```python
from build123d import *

# Parameters (mm, degrees)
BOSS_EXTRUDE1_DEPTH     = 0.8
CUT_EXTRUDE1_DEPTH      = 145.88389317
CUT_EXTRUDE2_DEPTH      = 145.88389317
MIRROR2_COPY_1_DEPTH    = 145.88389317
FILLET1_R               = 5
SKETCH4_R               = 3.65
BOSS_EXTRUDE4_DEPTH     = 3
CUT_EXTRUDE5_DEPTH      = 145.931509686
CUT_EXTRUDE5_DEPTH_BACK = 145.931509686
SKETCH2_4_R             = 1.8
CUT_EXTRUDE6_DEPTH      = 2.2
CUT_EXTRUDE6_DEPTH_BACK = 145.912740986
SKETCH4_4_R             = 2.85


with BuildPart() as part:
    # Sketch1 → Boss-Extrude1 (new body)
    with BuildSketch(Plane.XY):
        Polygon((85.45, 117), (-85.45, 117), (-85.45, 107.6), (-52.367829575, 50.3), (-85.45, -7), (-85.45, -15.5), (85.45, -15.5), (85.45, -7), (52.367829575, 50.3), (85.45, 107.6), align=None)
    extrude(amount=-BOSS_EXTRUDE1_DEPTH)

    # Sketch1_3 → Cut-Extrude1 (cut, through all)
    with BuildSketch(Plane.XY):
        Polygon((67.078361679, 85.779389009), (73.377429493, 96.689694505), (67.078361679, 107.6), (54.480226049, 107.6), (48.181158234, 96.689694505), (54.480226049, 85.779389009), align=None)
        Polygon((57.892542518, 69.869083514), (51.593474703, 80.779389009), (38.995339074, 80.779389009), (32.696271259, 69.869083514), (38.995339074, 58.958778018), (51.593474703, 58.958778018), align=None)
        Polygon((27.696271259, 69.869083514), (21.397203444, 80.779389009), (8.799067815, 80.779389009), (2.5, 69.869083514), (8.799067815, 58.958778018), (21.397203444, 58.958778018), align=None)
        Polygon((36.88209042, 85.779389009), (43.181158234, 96.689694505), (36.88209042, 107.6), (24.28395479, 107.6), (17.984886975, 96.689694505), (24.28395479, 85.779389009), align=None)
    cut_extrude1 = extrude(amount=-CUT_EXTRUDE1_DEPTH, mode=Mode.SUBTRACT)

    # Sketch1_4 → Cut-Extrude2 (cut, through all)
    with BuildSketch(Plane.XY):
        Polygon((-6.299067815, 107.6), (-12.598135629, 96.689694505), (-6.299067815, 85.779389009), (6.299067815, 85.779389009), (12.598135629, 96.689694505), (6.299067815, 107.6), align=None)
    cut_extrude2 = extrude(amount=-CUT_EXTRUDE2_DEPTH, mode=Mode.SUBTRACT)

    # Mirror1: Cut-Extrude1 across plane
    add(cut_extrude1.mirror(Plane(origin=(0, 0, 0), x_dir=(0, 0, 1), z_dir=(1, 0, 0))), mode=Mode.SUBTRACT)

    # Mirror2: Cut-Extrude1, Cut-Extrude2 across plane
    add(cut_extrude1.mirror(Plane(origin=(0, 50.3, 0), x_dir=(0, 0, 1), z_dir=(0, -1, 0))), mode=Mode.SUBTRACT)
    add(cut_extrude2.mirror(Plane(origin=(0, 50.3, 0), x_dir=(0, 0, 1), z_dir=(0, -1, 0))), mode=Mode.SUBTRACT)

    # Mirror2 copy 1 sketch → Mirror2 copy 1 (cut, through all)
    with BuildSketch(Plane(origin=(0, 100.6, 0), x_dir=(-1, 0, 0), z_dir=(0, 0, 1))):
        Polygon((67.078361679, 85.779389009), (73.377429493, 96.689694505), (67.078361679, 107.6), (54.480226049, 107.6), (48.181158234, 96.689694505), (54.480226049, 85.779389009), align=None)
        Polygon((57.892542518, 69.869083514), (51.593474703, 80.779389009), (38.995339074, 80.779389009), (32.696271259, 69.869083514), (38.995339074, 58.958778018), (51.593474703, 58.958778018), align=None)
        Polygon((27.696271259, 69.869083514), (21.397203444, 80.779389009), (8.799067815, 80.779389009), (2.5, 69.869083514), (8.799067815, 58.958778018), (21.397203444, 58.958778018), align=None)
        Polygon((36.88209042, 85.779389009), (43.181158234, 96.689694505), (36.88209042, 107.6), (24.28395479, 107.6), (17.984886975, 96.689694505), (24.28395479, 85.779389009), align=None)
    extrude(amount=-MIRROR2_COPY_1_DEPTH, mode=Mode.SUBTRACT)

    # Fillet1
    fillet1_edges = [part.edges().sort_by_distance(p)[0] for p in [
        (85.45, 117, -0.4),
        (-85.45, 117, -0.4),
        (-85.45, -15.5, -0.4),
        (85.45, -15.5, -0.4),
    ]]
    fillet(fillet1_edges, radius=FILLET1_R)

    # Sketch4 → Boss-Extrude4 (add)
    with BuildSketch(Plane.XY):
        with Locations(Location((-78, -11.829016319, 0), (0, 0, 180))):
            Circle(SKETCH4_R)
        with Locations(Location((78, 112.3, 0), (0, 0, 180))):
            Circle(SKETCH4_R)
    extrude(amount=BOSS_EXTRUDE4_DEPTH)

    # Sketch2_4 → Cut-Extrude5 (cut, two sides: drawn at the far end of the back side and taken through both)
    with BuildSketch(Plane(origin=(0, 0, -0.8), x_dir=(-1, 0, 0), z_dir=(0, 0, -1)).offset(-CUT_EXTRUDE5_DEPTH_BACK)):
        with Locations((-78, 112.3)):
            Circle(SKETCH2_4_R)
        with Locations((78, -11.829016319)):
            Circle(SKETCH2_4_R)
    extrude(amount=CUT_EXTRUDE5_DEPTH + CUT_EXTRUDE5_DEPTH_BACK, mode=Mode.SUBTRACT)

    # Sketch4_4 → Cut-Extrude6 (cut, two sides: drawn at the far end of the back side and taken through both)
    with BuildSketch(Plane.XY.offset(-CUT_EXTRUDE6_DEPTH_BACK)):
        with Locations((-78, -11.829016319)):
            Circle(SKETCH4_4_R)
        with Locations((78, 112.3)):
            Circle(SKETCH4_4_R)
    extrude(amount=CUT_EXTRUDE6_DEPTH + CUT_EXTRUDE6_DEPTH_BACK, mode=Mode.SUBTRACT)


solid = part.part
```
Geometry check sheet. Reference: the model listing, model coordinates, mm. A direction names the side the tool comes from. Give positions to 0.01 mm unless a question says otherwise; leave off trailing zeros. Write each loop counter-clockwise with the first axis right and the second up, starting at its lowest first coordinate (ties: lowest second). Pieces come first, ordered by that corner, then holes. Notation, with made-up numbers: (29.5, 30) -> (41.5, 30) arc R27 ccw to (41.5, 60) -> close; hole circle Ø6 at (59, 39). An arc over 180 degrees is marked (long way). Use one line per item in the form item = value.
Item 1: Sectioned sample at D-D on x = 78. Enter the section's corners in (y, z).
Results list:
outline = (-15.5, -0.8) -> (5.9, -0.8) -> (5.9, 0) -> (-15.5, 0) -> close; (94.7, -0.8) -> (109.45, -0.8) -> (109.45, 2.2) -> (110.5, 2.2) -> (110.5, 3) -> (108.65, 3) -> (108.65, 0) -> (94.7, 0) -> close; (114.1, 2.2) -> (115.15, 2.2) -> (115.15, -0.8) -> (117, -0.8) -> (117, 0) -> (115.95, 0) -> (115.95, 3) -> (114.1, 3) -> close
Item 2: Mould release check, pull along Y, two halves, no side actions. Record for faces 1 (the flat face through (35.89, 25.2, -0.39)), 2 (the cylindrical face through (83.95, 115.57, -0.41)): released by +Y, released by -Y, zero draft, split by the parting line, or undercut.
Results list:
face_1 = undercut
face_2 = released by +Y
Item 3: Sectioned sample at B-B on y = 88. Enter the section's corners in (x, z), plus the area to 3 significant figures.
Results list:
outline = (-74.13, -0.8) -> (-68.36, -0.8) -> (-68.36, 0) -> (-74.13, 0) -> close; (-53.2, -0.8) -> (-38.16, -0.8) -> (-38.16, 0) -> (-53.2, 0) -> close; (-23, -0.8) -> (-7.58, -0.8) -> (-7.58, 0) -> (-23, 0) -> close; (7.58, -0.8) -> (23, -0.8) -> (23, 0) -> (7.58, 0) -> close; (38.16, -0.8) -> (53.2, -0.8) -> (53.2, 0) -> (38.16, 0) -> close; (68.36, -0.8) -> (74.13, -0.8) -> (74.13, 0) -> (68.36, 0) -> close
area = 58.0 mm2
Item 4: Sectioned sample at A-A on x = 60. Enter the section's corners in (y, z), plus the area to 3 significant figures.
Results list:
outline = (-15.5, -0.8) -> (-7, -0.8) -> (-7, 0) -> (-15.5, 0) -> close; (14.82, -0.8) -> (37.08, -0.8) -> (37.08, 0) -> (14.82, 0) -> close; (63.52, -0.8) -> (85.78, -0.8) -> (85.78, 0) -> (63.52, 0) -> close; (107.6, -0.8) -> (117, -0.8) -> (117, 0) -> (107.6, 0) -> close
area = 49.9 mm2
Item 5: Depth check by flat-ended pin: pin 1 Ø3 at (x, y) = (-78, -11.83) entering from -Z; pin 2 Ø8 at (x, y) = (-7.5, 91.5) entering from +Z; pin 3 Ø1 at (y, z) = (97.5, 0) entering from +X. Enter the tip coordinate at first touch or a pass-through.
Results list:
pin_1 = through
pin_2 = 0
pin_3 = 79.91
Item 6: Scan lines: line 1 (Y direction, x = 48, z = -0.05); line 2 (X direction, y = 32, z = -0.15); line 3 (Y direction, x = 78, z = 2.75). Record each from-to range of solid material in increasing order.
Results list:
line_1 = -15.5 to 19.82, 41.64 to 58.96, 80.78 to 117
line_2 = -62.93 to -57.16, -33.43 to -26.96, -3.23 to 3.23, 26.96 to 33.43, 57.16 to 62.93
line_3 = 108.65 to 110.5, 114.1 to 115.95
Item 7: Sectioned sample at C-C on z = 1.6. Enter the section's corners in (x, y), plus the area to 3 significant figures.
Results list:
outline = circle Ø7.3 at (-78, -11.83); circle Ø7.3 at (78, 112.3); hole circle Ø5.7 at (-78, -11.83); hole circle Ø5.7 at (78, 112.3)
area = 32.7 mm2
Item 8: Access from +Z, -Z, +X, -X, +Y, -Y to the whole of each face (thin tool, end or side, straight path). Record for faces 3 (the flat face through (21.18, 102.22, -0.39)), 4 (the flat face through (-68.68, 22.05, -0.39)), 5 (the flat face through (78, 110, 2.2)).
Results list:
face_3 = +Z, -Z
face_4 = +Z, -Z, -X
face_5 = -Z
